Could you check a few things on this model? Use its own coordinates, in mm. A direction names the side the tool comes from. Give positions to 0.01 mm unless a question says otherwise; leave off trailing zeros. Order: outer loops, then holes, each group sorted by start corner. A loop starts at its lowest first (then second) coordinate and runs counter-clockwise, first axis right, second up. Notation, with made-up numbers: M 22,83.5 L 34,83.5 A15 cw 34,97.5 Z; hole C -31,-13.75 d5. An arc over 180 degrees is marked long. Return JSON: item names as keys, results as strings. Group by question number.
Autodesk Inventor part; units mm, degrees
ref_plane "Work Plane1" through (7, 0, 0) normal (-1, 0, 0) x (0, 0, 1)
ref_plane "YZ Plane" through (0, 0, 0) normal (1, 0, 0) x (0, 1, 0)
ref_plane "XZ Plane" through (0, 0, 0) normal (0, 1, 0) x (-1, 0, 0)
sketch "Sketch1" plane through (0, 0, 0) normal (0, 1, 0) x (-1, 0, 0)
  point P0 (0, 0)
sketch "Sketch2" plane through (0, 0, 0) normal (1, 0, 0) x (0, 1, 0)
  point P0 (0, 0)
sketch "Sketch3" plane through (0, 0, 0) normal (1, 0, 0) x (0, 1, 0)
  line L0 (0, 0) -> (0.5, 0)
  line L1 (0.5, 0) -> (0.5, 1)
  line L2 (0.5, 1) -> (0, 1)
  line L3 (0, 1) -> (0, 0)
  dimension "d0" = 0.5
  dimension "d1" = 1
extrude "Extrusion1" add sketch "Sketch3" along normal blind 9
sketch "Sketch4" plane through (9, 0, 0) normal (1, 0, 0) x (0, 0, -1)
  line L0 (0, 0) -> (0, 0.5)
  circle A0 centre (0.75, 0.25) radius 0.375
  line L1 (0, 0.5) -> (-1, 0.5)
  line L2 (-1, 0.5) -> (-1, 0) construction
  line L3 (-1, 0.25) -> (1.9779, 0.25) construction
  line L4 (0, 0) -> (0, 0.5)
  line L5 (0, 0.5) -> (-1, 0.5)
  line L6 (-1, 0.5) -> (-1, 0)
  line L7 (-1, 0) -> (0, 0)
  line L8 (-1, 0) -> (0, 0)
  line L9 (-1, 0.5) -> (0.3417, 1.1256)
  line L10 (-1, 0) -> (0.3417, -0.6256)
  arc A1 (0.3417, -0.6256) -> (0.3417, 1.1256) centre (0.75, 0.25) ccw
  point P0 (-0.5, 0)
  dimension "d9" = 0.75
  dimension "d12" = 1.25
  dimension "d13" = 0
  dimension "d14" = 25
extrude "Extrusion2" add sketch "Sketch4" against normal blind 1 contours L0 L1 L9 A1 L10 L7
ref_plane "Work Plane1" through (7, 0, 0) normal (-1, 0, 0) x (0, 0, 1)
sketch "Sketch5" plane through (7, 0, 0) normal (-1, 0, 0) x (0, 0, 1)
  line L0 (-0.3417, -0.6256) -> (1, 0)
  line L1 (0, 0) -> (1, 0)
  line L2 (0, 0.5) -> (0, 0)
  line L3 (1, 0.5) -> (0, 0.5)
  line L4 (1, 0.5) -> (-0.3417, 1.1256)
  arc A0 (-0.3417, 1.1256) -> (-0.3417, -0.6256) centre (-0.75, 0.25) ccw
  circle A1 centre (-0.75, 0.25) radius 0.375
extrude "Extrusion3" add sketch "Sketch5" along normal blind 0.75
sketch "Sketch6" plane through (6.25, 0, 0) normal (-1, 0, 0) x (0, 0, 1)
  circle A0 centre (-0.75, 0.25) radius 0.375
  point P0 (0, 0)
extrude "Extrusion4" add sketch "Sketch6" against normal blind 0.05
sketch "Sketch7" plane through (0, 0.5, 1) normal (0, 1, 0) x (1, 0, 0)
  line L0 (8, 2.6833) -> (9, 2.6833)
  line L1 (9, 2.6833) -> (9, 2.0295)
  line L2 (9, 2.0295) -> (8, 2.0295)
  line L3 (8, 2.0295) -> (8, 2.6833)
  line L4 (9, 0) -> (8, 0)
  line L5 (8, 0) -> (8, 1)
  line L6 (8, 1) -> (8, 1.4705)
  line L7 (8, 1.4705) -> (9, 1.4705)
  line L8 (9, 1.4705) -> (9, 0)
  line L9 (8, 0) -> (7, 0)
  line L10 (7, 1) -> (7, 0)
  line L11 (7, 1.4705) -> (7, 1)
  line L12 (6.3, 1.4705) -> (7, 1.4705)
  line L13 (6.3, 2.0295) -> (6.3, 1.4705)
  line L14 (7, 2.0295) -> (6.3, 2.0295)
  line L15 (7, 2.6833) -> (7, 2.0295)
  line L16 (6.25, 2.6833) -> (7, 2.6833)
  line L17 (6.25, 1) -> (6.25, 2.6833)
  line L18 (0, 1) -> (6.25, 1)
  line L19 (0, 0) -> (0, 1)
  line L20 (6.25, 0) -> (0, 0)
  line L21 (7, 0) -> (6.25, 0)
  line L22 (7, 1) -> (8, 1)
  line L23 (6.25, 0) -> (6.25, 1)
  circle A0 centre (7.5, 0.5) radius 0.5
  line L24 (7, 0) -> (8, 0)
  line L25 (7, 0) -> (7, 1.3417)
  line L26 (7, 1) -> (8, 1)
  line L27 (8, 0) -> (8, 1.3417)
  circle A1 centre (7.5, 0.5) radius 0.125
  line L28 (7, 0) -> (7.4116, 0.4116)
  line L29 (7.5884, 0.5884) -> (8, 1)
  line L30 (7, 1) -> (7.4116, 0.5884)
  line L31 (7.5884, 0.4116) -> (8, 0)
  dimension "d22" = 0.25
extrude "Extrusion5" cut sketch "Sketch7" against normal through all contours A1
sketch "Sketch8" plane through (0, 0.5, 1) normal (0, 1, 0) x (1, 0, 0)
  line L0 (0, 1) -> (6.25, 1)
  line L1 (0, 0) -> (1, 0)
  line L2 (1, 0) -> (1, 1)
  line L3 (1, 1) -> (0, 1)
  line L4 (0, 1) -> (0, 0)
  line L5 (0, 1) -> (0, 0)
  circle A0 centre (0.5, 0.5) radius 0.25
  line L6 (0, 0) -> (0.3232, 0.3232)
  line L7 (0.6768, 0.6768) -> (1, 1)
  line L8 (0, 1) -> (0.3232, 0.6768)
  line L9 (0.6768, 0.3232) -> (1, 0)
  dimension "d25" = 1
  dimension "d26" = 0.5
extrude "Extrusion6" cut sketch "Sketch8" against normal through all contours A0
properties part number "rocker"
1. Imagine slicing it at D-D, the plane x = 8.25. Please give me the cut outline in (y, z) (3 decimals), plus the area to 3 significant figures.
2. Imagine slicing it at B-B, the plane y = 0.25. Please give me the cut outline in (x, z) (3 decimals), plus the area to 3 significant figures.
3. For pin 1 (0.8 mm diameter, centred on x = 3, z = 0.5, fed in from +Y); pin 2 (0.5 mm diameter, centred on x = 7.5, z = 0.5, fed in from -Y); pin 3 (0.6 mm diameter, centred on x = 7.5, y = 0.5, fed in from -Z), each with a flat end and sliding along its axis, tell me the tip position at first contact or that it passes through.
4. I need wall thicknesses on L1, parallel to X at y = 0.3, z = 0.5 (3 decimals); L2, parallel to Y at x = 6.6, z = -0.75 (3 decimals); L3, parallel to X at y = -0.4, z = -1.3. Which ranges of each line are inside material? Lowest first, please. Write a range as from..to.
5. Which directions (+Z, -Z, +X, -X, +Y, -Y) give clear straight access to the entire face, cutting with the end or side of a thin tool? Please do faces 1 (the flat face through (3.1, 0, 0.5)), 2 (the flat face through (8.507, 0.808, 0.339)).
6. Imagine slicing it at C-C, the plane z = -0.75. Please give me the cut outline in (x, y) (3 decimals), plus the area to 3 significant figures.
7. If we mould it in two halves opening along X, with no side actions, what happens to faces 3 (the flat face through (3.1, 0.5, 0.5)), 4 (the flat face through (8, 1, -1)), 5 (the flat face through (9, 0, 0)), 6 (the flat face through (7, 1, -1))? For each: pulls with the +X half, pulls with the -X half, needs draft (parallel to the pull), parting line crosses it, or undercut.
8. Imagine slicing it at A-A, the plane x = 0.5. Please give me the cut outline in (y, z), plus the area to 3 significant figures.
Values:
{
 "1": {"outline": "M -0.626,-0.342 A0.966 ccw long 1.126,-0.342 L 0.5,1 L 0,1 Z; hole C 0.25,-0.75 d0.75", "area": "3.30 mm²"},
 "2": {"outline": "M 0,0 L 6.25,0 L 6.25,-1.716 L 7,-1.716 L 7,-1.125 L 6.3,-1.125 L 6.3,-0.375 L 7,-0.375 L 7,0 L 8,0 L 8,-0.375 L 9,-0.375 L 9,1 L 0,1 Z; M 8,-1.716 L 9,-1.716 L 9,-1.125 L 8,-1.125 Z; hole C 0.5,0.5 d0.5; hole C 7.5,0.5 d0.25", "area": "10.5 mm²"},
 "3": {"pin 1": "stops at y = 0.5", "pin 2": "stops at y = 0", "pin 3": "stops at z = 0"},
 "4": {"L1": "x = 0..0.25, 0.75..7.375, 7.625..9", "L2": "y = -0.716..-0.125, 0.625..1.216", "L3": "x = 6.25..7, 8..9"},
 "5": {"face 1": "+Z, -Z, -X, -Y", "face 2": "+Z, +X, -X, +Y"},
 "6": {"outline": "M 6.25,-0.716 L 7,-0.716 L 7,-0.125 L 6.3,-0.125 L 6.3,0.625 L 7,0.625 L 7,1.216 L 6.25,1.216 Z; M 8,-0.716 L 9,-0.716 L 9,-0.125 L 8,-0.125 Z; M 8,0.625 L 9,0.625 L 9,1.216 L 8,1.216 Z", "area": "2.11 mm²"},
 "7": {"face 3": "needs draft", "face 4": "undercut", "face 5": "pulls with the +X half", "face 6": "undercut"},
 "8": {"outline": "M 0,0 L 0.5,0 L 0.5,0.25 L 0,0.25 Z; M 0,0.75 L 0.5,0.75 L 0.5,1 L 0,1 Z", "area": "0.250 mm²"}
}
